The listing builds one solid part. Answer for the finished solid, in the listing's coordinates (mm). A direction names the side the tool comes from. Round coordinates to 2 decimals unless told otherwise and drop trailing zeros. Order: outer loops, then holes, each group sorted by start corner. A loop starts at its lowest first (then second) coordinate and runs counter-clockwise, first axis right, second up. Notation, with made-up numbers: (-8, 82.5) - (2, 82.5) arc R28 cw to (2, 107.5) - close; hole circle Ø11 at (61, 39.5). An arc over 180 degrees is marked (long way). One line per item, written item: value. Start each with the question number.
1. Flat-ended cylindrical pins translate along their axes: P1, Ø10, axis at x = 14.5, y = 23.5, coming from the -Z side; P2, Ø3, axis at x = -0.5, z = 4, coming from the -Y side; P3, Ø1.1, axis at x = 13, z = 3, coming from the +Y side; P4, Ø0.8, axis at y = 22, z = 2.5, coming from the -X side. Find the tip coordinate at first contact, or state that the pin passes through.
2. Section A-A, the plane z = 2.6 is taken. Give the vertices of the cut face in (x, y).
3. Straight lines are drawn through the part: line 1 (Y direction, x = 0, z = 3.1); line 2 (Y direction, x = 3, z = 1); line 3 (X direction, y = 0, z = 4.2). For each, find the intervals that lie inside material, in ascending order.
4. A tool of negligible diameter and unlimited length cuts with its end or side. For faces 4 (the flat face through (0, -6.2, 1)), 5 (the flat face through (-3.2, 20, 1)), 6 (the flat face through (-4.7, 23, 3)), 7 (the cylindrical face through (-7.451, 12.322, 3.226)), 8 (the cylindrical face through (15.783, -0.051, 3.226)), from which of +Z, -Z, +X, -X, +Y, -Y can it reach the whole face along a straight path? Write none if from no direction.
5. Section D-D, the plane y = 17 is taken. Give the vertices of the cut face in (x, z), then the cut area to 3 significant figures.
6. For a pull along Y with two mould halves and no side action, classify faces 1 (the flat face through (-20, 4, 1)), 2 (the flat face through (3.2, 20, 1)), 3 (the flat face through (0, -13.2, 1)) as released by +Y, released by -Y, zero draft, split by the parting line, or undercut.
7. Section C-C, the plane x = 0 is taken. Give the vertices of the cut face in (y, z), then the cut area to 3 significant figures.
8. Section B-B, the plane y = 0 is taken. Give the vertices of the cut face in (x, z), then the cut area to 3 significant figures.
from build123d import *

# Parameters (mm, degrees)
CROQUIS1_W                  = 40
CROQUIS1_H                  = 45
CROQUIS1_W_2                = 6.4
CROQUIS1_H_2                = 11.3
SALIENTE_EXTRUIR1_DEPTH     = 1.5
REDONDEO1_R                 = 10
EXTRUIR_L_MINA1_OUTLINE_W   = 9.4
EXTRUIR_L_MINA1_OUTLINE_H   = 6.3
EXTRUIR_L_MINA1_OUTLINE_W_2 = 6.4
EXTRUIR_L_MINA1_OUTLINE_H_2 = 3.3
EXTRUIR_L_MINA1_DEPTH       = 4
EXTRUIR_L_MINA3_DEPTH       = 5
CROQUIS1_10_W               = 6.4
CROQUIS1_10_H               = 8
CORTAR_EXTRUIR5_DEPTH       = 1.5


# Read off the part's stored shape, not the designer's step: Extruir-Lámina1
with BuildPart() as part:
    # Croquis1 → Saliente-Extruir1 (new body)
    with BuildSketch(Plane.XY):
        with Locations((0, 9.3)):
            Rectangle(CROQUIS1_W, CROQUIS1_H)
        with BuildLine():
            Line((3.660601044, -6.2), (-3.660601044, -6.2))
            ThreePointArc((-3.660601044, -6.2), (-7.2, 0), (-3.660601044, 6.2))
            Line((-3.660601044, 6.2), (3.660601044, 6.2))
            ThreePointArc((3.660601044, 6.2), (7.2, 0), (3.660601044, -6.2))
        make_face(mode=Mode.SUBTRACT)
        with Locations((0, 18.85)):
            Rectangle(CROQUIS1_W_2, CROQUIS1_H_2, mode=Mode.SUBTRACT)
    extrude(amount=SALIENTE_EXTRUIR1_DEPTH)

    # Redondeo1
    redondeo1_edges = [part.edges().sort_by_distance(p)[0] for p in [
        (-20, 31.8, 0.75),
        (20, 31.8, 0.75),
    ]]
    fillet(redondeo1_edges, radius=REDONDEO1_R)

    # Extruir-Lámina1 outline → Extruir-Lámina1 (add)
    with BuildSketch(Plane.XY):
        with Locations((0, 22.85)):
            Rectangle(EXTRUIR_L_MINA1_OUTLINE_W, EXTRUIR_L_MINA1_OUTLINE_H)
        with Locations((0, 22.85)):
            Rectangle(EXTRUIR_L_MINA1_OUTLINE_W_2, EXTRUIR_L_MINA1_OUTLINE_H_2, mode=Mode.SUBTRACT)
    extrude(amount=EXTRUIR_L_MINA1_DEPTH)

    # Croquis1<11> → Extruir-Lámina3 (add)
    with BuildSketch(Plane.XY):
        with BuildLine():
            ThreePointArc((-8.140559831, -10.007061788), (-6.473500548, 11.158126664), (12.727922061, 2.1))
            Line((12.727922061, 2.1), (14.127922061, 2.1))
            ThreePointArc((14.127922061, 2.1), (14.283143274, 0), (14.127922061, -2.1))
            Line((14.127922061, -2.1), (12.727922061, -2.1))
            ThreePointArc((12.727922061, -2.1), (11.158126664, -6.473500548), (8.140559831, -10.007061788))
            Line((8.140559831, -10.007061788), (9.087136556, -11.170673624))
            ThreePointArc((9.087136556, -11.170673624), (12.121162438, -7.774150831), (13.942740046, -3.6))
            Line((13.942740046, -3.6), (15.367095093, -3.6))
            ThreePointArc((15.367095093, -3.6), (15.783143274, 0), (15.367095093, 3.6))
            Line((15.367095093, 3.6), (13.942740046, 3.6))
            ThreePointArc((13.942740046, 3.6), (-7.774150831, 12.121162438), (-9.087136556, -11.170673624))
            Line((-9.087136556, -11.170673624), (-8.140559831, -10.007061788))
        make_face()
    extrude(amount=EXTRUIR_L_MINA3_DEPTH)

    # Croquis1<10> → Cortar-Extruir5 (cut)
    with BuildSketch(Plane.XY):
        with Locations((0, 17.2)):
            Rectangle(CROQUIS1_10_W, CROQUIS1_10_H)
    extrude(amount=CORTAR_EXTRUIR5_DEPTH, mode=Mode.SUBTRACT)


solid = part.part
Answer list:
1. P1: stops at z = 0
1. P2: stops at y = 12.74
1. P3: stops at y = 7.24
1. P4: stops at x = -4.7
2. outline: (-9.09, -11.17) - (-8.14, -10.01) arc R12.9 cw (long way) to (12.73, 2.1) - (14.13, 2.1) arc R14.28 cw to (14.13, -2.1) - (12.73, -2.1) arc R12.9 cw to (8.14, -10.01) - (9.09, -11.17) arc R14.4 ccw to (13.94, -3.6) - (15.37, -3.6) arc R15.78 ccw to (15.37, 3.6) - (13.94, 3.6) arc R14.4 ccw (long way) to start; (-4.7, 19.7) - (4.7, 19.7) - (4.7, 26) - (-4.7, 26) - close; hole (-3.2, 21.2) - (3.2, 21.2) - (3.2, 24.5) - (-3.2, 24.5) - close
3. line 1: y = 12.9 to 14.4, 19.7 to 21.2, 24.5 to 26
3. line 2: y = -13.2 to -6.2, 6.2 to 13.2, 24.5 to 31.8
3. line 3: x = -14.4 to -12.9, 14.28 to 15.78
4. face 4: +Z, -Z
4. face 5: -Z
4. face 6: +Z, -X, +Y
4. face 7: +Z
4. face 8: +Z, +X
5. outline: (-20, 0) - (-3.2, 0) - (-3.2, 1.5) - (-20, 1.5) - close; (3.2, 0) - (20, 0) - (20, 1.5) - (3.2, 1.5) - close
5. area: 50.4 mm²
6. face 1: zero draft
6. face 2: undercut
6. face 3: released by -Y
7. outline: (-13.2, 0) - (-6.2, 0) - (-6.2, 1.5) - (-13.2, 1.5) - close; (6.2, 0) - (13.2, 0) - (13.2, 1.5) - (14.4, 1.5) - (14.4, 5) - (12.9, 5) - (12.9, 1.5) - (6.2, 1.5) - close; (19.7, 1.5) - (21.2, 1.5) - (21.2, 4) - (19.7, 4) - close; (24.5, 0) - (31.8, 0) - (31.8, 1.5) - (26, 1.5) - (26, 4) - (24.5, 4) - close
7. area: 44.7 mm²
8. outline: (-20, 0) - (-7.2, 0) - (-7.2, 1.5) - (-12.9, 1.5) - (-12.9, 5) - (-14.4, 5) - (-14.4, 1.5) - (-20, 1.5) - close; (7.2, 0) - (20, 0) - (20, 1.5) - (15.78, 1.5) - (15.78, 5) - (14.28, 5) - (14.28, 1.5) - (7.2, 1.5) - close
8. area: 48.9 mm²
